Can you work these out from the model? Positions are in its coordinate system, mm. Face numbers are marked on the shaded views. A direction names the side the tool comes from. Coordinates: 2 decimals unless noted, no trailing zeros. Loops run counter-clockwise (first coordinate to the right, second up) from the corner with the lowest first, then second, coordinate; pieces in that order, holes last.
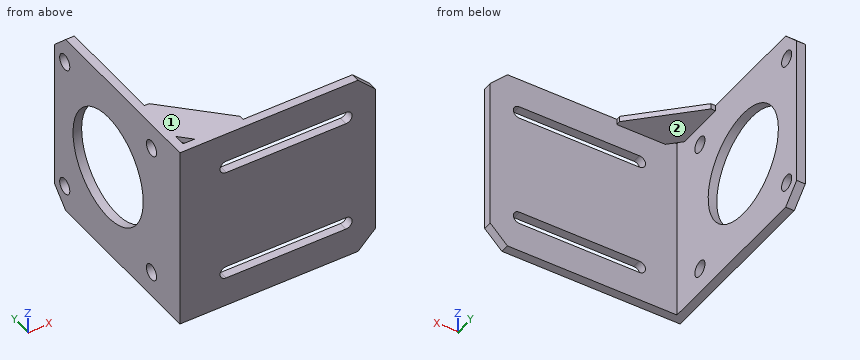
```python
from build123d import *

# Parameters (mm, degrees)
BOSS_EXTRUDE1_DEPTH = 65
CHAMFER1_SIZE       = 6
BOSS_EXTRUDE2_DEPTH = 2
SKETCH3_R           = 19.05
SKETCH3_R_2         = 2.75
CUT_EXTRUDE1_DEPTH  = 3
CUT_EXTRUDE2_DEPTH  = 3


with BuildPart() as part:
    # Sketch1 → Boss-Extrude1 (new body)
    with BuildSketch(Plane.XY):
        Polygon((0, 0), (0, 68), (3, 68), (3, 3), (68, 3), (68, 0), align=None)
    extrude(amount=BOSS_EXTRUDE1_DEPTH)

    # Chamfer1
    chamfer1_edges = [part.edges().sort_by_distance(p)[0] for p in [
        (1.5, 68, 65),
        (1.5, 68, 0),
        (68, 1.5, 65),
        (68, 1.5, 0),
    ]]
    chamfer(chamfer1_edges, length=CHAMFER1_SIZE)

    # Sketch2 → Boss-Extrude2 (add)
    with BuildSketch(Plane.XY.offset(65)):
        Polygon((4.600185007, 23.955878092), (23.955878092, 4.600185007), (23.955878092, 3), (7.047822016, 3), (3, 7.047822016), (3, 23.955878092), align=None)
    extrude(amount=-BOSS_EXTRUDE2_DEPTH)

    # Sketch3 → Cut-Extrude1 (cut)
    with BuildSketch(Plane.ZY):
        with Locations((32.5, 39)):
            Circle(SKETCH3_R)
        with Locations((8.95, 62.55)):
            Circle(SKETCH3_R_2)
        with Locations((56.05, 62.55)):
            Circle(SKETCH3_R_2)
        with Locations((8.95, 15.45)):
            Circle(SKETCH3_R_2)
        with Locations((56.05, 15.45)):
            Circle(SKETCH3_R_2)
    extrude(amount=-CUT_EXTRUDE1_DEPTH, mode=Mode.SUBTRACT)

    # Sketch4 → Cut-Extrude2 (cut)
    with BuildSketch(Plane.XZ):
        with BuildLine():
            Line((16.1, 54.65), (57.8, 54.65))
            ThreePointArc((57.8, 54.65), (59.95, 52.5), (57.8, 50.35))
            Line((57.8, 50.35), (16.1, 50.35))
            ThreePointArc((16.1, 50.35), (13.95, 52.5), (16.1, 54.65))
        make_face()
        with BuildLine():
            Line((16.1, 14.65), (57.8, 14.65))
            ThreePointArc((57.8, 14.65), (59.95, 12.5), (57.8, 10.35))
            Line((57.8, 10.35), (16.1, 10.35))
            ThreePointArc((16.1, 10.35), (13.95, 12.5), (16.1, 14.65))
        make_face()
    extrude(amount=-CUT_EXTRUDE2_DEPTH, mode=Mode.SUBTRACT)


solid = part.part
```
Item 1: Suppose I cut it at C-C, the plane z = 56.05. Please give me the cut outline in (x, y).
Results are:
outline: (0, 0) - (68, 0) - (68, 3) - (3, 3) - (3, 12.7) - (0, 12.7) - close; (0, 18.2) - (3, 18.2) - (3, 59.8) - (0, 59.8) - close; (0, 65.3) - (3, 65.3) - (3, 68) - (0, 68) - close
Item 2: Suppose I cut it at D-D, the plane y = 31.5. Please give me the cut outline in (x, z), plus the area to 3 significant figures.
Results are:
outline: (0, 0) - (3, 0) - (3, 14.99) - (0, 14.99) - close; (0, 50.01) - (3, 50.01) - (3, 65) - (0, 65) - close
area: 89.9 mm2
Item 3: Suppose I cut it at A-A, the plane z = 32.5. Please give me the cut outline in (x, y), plus the area to 3 significant figures.
Results are:
outline: (0, 0) - (68, 0) - (68, 3) - (3, 3) - (3, 19.95) - (0, 19.95) - close; (0, 58.05) - (3, 58.05) - (3, 68) - (0, 68) - close
area: 285 mm2
Item 4: I need wall thicknesses on line 1 along Y through (x, z) = (1, 56); line 2 along Y through (x, z) = (1.1, 32.5); line 3 along X through (y, z) = (17.5, 36.5). Which ranges of each line are inside material? Lowest first, please.
Results are:
line 1: y = 0 to 12.7, 18.2 to 59.8, 65.3 to 68
line 2: y = 0 to 19.95, 58.05 to 68
line 3: x = 0 to 3
Item 5: On a 3-axis mill with a long thin cutter (end or side, diameter ignored), from which of +Z, -Z, +X, -X, +Y, -Y can I reach the whole of each face in a straight line? I mean the marked faces 1 and 2. Say none if no direction works.
Results are:
face 1: +Z, +X, -X, +Y, -Y
face 2: -Z, +X, +Y
Item 6: I'm going to push flat-ended pins straight in: P1, Ø10, axis at y = 10, z = 21, coming from the -X side; P2, Ø8, axis at y = 57, z = 18, coming from the +X side; P3, Ø0.8, axis at x = 4, z = 64, coming from the +Y side; P4, Ø12, axis at x = 18, z = 50, coming from the +Y side. Where does each tip first touch, or does it pass through?
Results are:
P1: stops at x = 0
P2: stops at x = 3
P3: stops at y = 23.96
P4: stops at y = 3
Item 7: Suppose I cut it at B-B, the plane x = 42. Please give me the cut outline in (y, z).
Results are:
outline: (0, 0) - (3, 0) - (3, 10.35) - (0, 10.35) - close; (0, 14.65) - (3, 14.65) - (3, 50.35) - (0, 50.35) - close; (0, 54.65) - (3, 54.65) - (3, 65) - (0, 65) - close
